Geometry check sheet. Reference: the model listing, model coordinates, mm. Face numbers are marked on the shaded views. A direction names the side the tool comes from. Round coordinates to 2 decimals unless told otherwise and drop trailing zeros. Loops run counter-clockwise (first coordinate to the right, second up) from the corner with the lowest first, then second, coordinate; pieces in that order, holes last. Notation, with made-up numbers: (49, -1) -> (108, -1) arc R26 cw to (108, 15) -> close; hole circle Ø6 at (13.5, 63). An arc over 180 degrees is marked (long way). Use one line per item in the form item = value.
from build123d import *

# Parameters (mm, degrees)
SKETCH2_R            = 10.16
BOSS_EXTRUDE1_DEPTH  = 10.16
SKETCH3_R            = 9.525
BOSS_EXTRUDE2_DEPTH  = 129.54
SKETCH4_R            = 6.35
BOSS_EXTRUDE4_DEPTH  = 63.5
SKETCH5_R            = 3.175
BOSS_EXTRUDE5_DEPTH  = 6.35
SKETCH8_W            = 1.27
SKETCH8_H            = 2.54
EXTRUDE_THIN1_DEPTH  = 8.89
SKETCH9_W            = 7.62
SKETCH9_H            = 5.08
BOSS_EXTRUDE14_DEPTH = 5.08


with BuildPart() as part:
    # Sketch2 → Boss-Extrude1 (new body)
    with BuildSketch(Plane.XY):
        Circle(SKETCH2_R)
    extrude(amount=BOSS_EXTRUDE1_DEPTH)

    # Sketch3 → Boss-Extrude2 (add)
    with BuildSketch(Plane.XY.offset(10.16)):
        Circle(SKETCH3_R)
    extrude(amount=BOSS_EXTRUDE2_DEPTH)

    # Sketch4 → Boss-Extrude4 (add)
    with BuildSketch(Plane.XY.offset(139.7)):
        Circle(SKETCH4_R)
    extrude(amount=BOSS_EXTRUDE4_DEPTH)

    # Sketch5 → Boss-Extrude5 (add)
    with BuildSketch(Plane.XY.offset(203.2)):
        Circle(SKETCH5_R)
    extrude(amount=BOSS_EXTRUDE5_DEPTH)

    # Sketch8 → Extrude-Thin1 (add)
    with BuildSketch(Plane(origin=(0, 2.54, 0), x_dir=(1, 0, 0), z_dir=(0, 1, 0))):
        with Locations((-1.397, -25.185428327)):
            Rectangle(SKETCH8_W, SKETCH8_H)
        with Locations((1.397, -25.185428327)):
            Rectangle(SKETCH8_W, SKETCH8_H)
    extrude(amount=EXTRUDE_THIN1_DEPTH)

    # Sketch9 → Boss-Extrude14 (add)
    with BuildSketch(Plane(origin=(0, 11.43, 0), x_dir=(1, 0, 0), z_dir=(0, 1, 0))):
        with Locations((0, -25.964513942)):
            Rectangle(SKETCH9_W, SKETCH9_H)
    extrude(amount=BOSS_EXTRUDE14_DEPTH)


solid = part.part
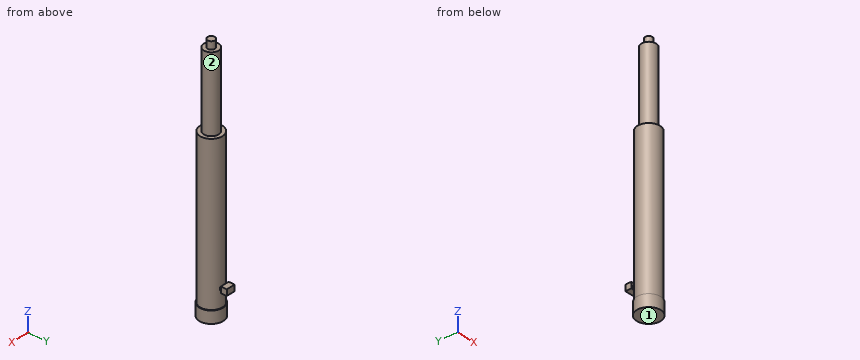
1. Material ranges on line 1 along Z through (x, y) = (-2, 5.5); line 2 along Z through (x, y) = (-8, -3.75); line 3 along Y through (x, z) = (-0.5, 74), recorded low to high.
Return value:
line_1 = 0 to 203.2
line_2 = 0 to 139.7
line_3 = -9.51 to 9.51
2. Section check A-A (y = 0). Record the boundary of the cut face in (x, z) (3 decimals).
Return value:
outline = (-10.16, 0) -> (10.16, 0) -> (10.16, 10.16) -> (9.525, 10.16) -> (9.525, 139.7) -> (6.35, 139.7) -> (6.35, 203.2) -> (3.175, 203.2) -> (3.175, 209.55) -> (-3.175, 209.55) -> (-3.175, 203.2) -> (-6.35, 203.2) -> (-6.35, 139.7) -> (-9.525, 139.7) -> (-9.525, 10.16) -> (-10.16, 10.16) -> close
3. Tool access check on the marked faces 1 and 2. Record the directions out of +Z, -Z, +X, -X, +Y, -Y that give a thin tool (end or side, any length) a straight path to the whole face; none if there is none.
Return value:
face_1 = -Z, +X, -X, +Y, -Y
face_2 = +Z
4. Gauge pin test, flat ends, axial feed: pin 1 (1 mm diameter, centred on x = -5.5, y = -0.5, fed in from +Z); pin 2 (2.5 mm diameter, centred on y = 15, z = 26, fed in from +X); pin 3 (8 mm diameter, centred on x = -3.5, z = 169.5, fed in from -Y). Record the tip position at first contact, or that the pin passes through.
Return value:
pin_1 = 203.2
pin_2 = 3.81
pin_3 = -6.35
5. Section check B-B (z = 86.5). Record the boundary of the cut face in (x, y) (3 decimals).
Return value:
outline = circle Ø19.05 at (0, 0)
